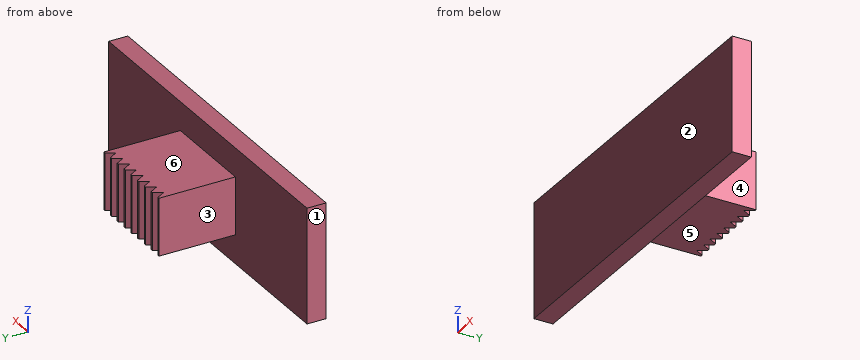
from build123d import *

# Parameters (mm, degrees)
SKETCH1_W           = 18
SKETCH1_H           = 6
BOSS_EXTRUDE1_DEPTH = 1
SKETCH2_W           = 5
SKETCH2_H           = 3
BOSS_EXTRUDE2_DEPTH = 4
CUT_EXTRUDE1_START  = -5.5
CUT_EXTRUDE1_DEPTH  = 8
LPATTERN1_COUNT     = 8
LPATTERN1_PITCH     = 0.614285714


with BuildPart() as part:
    # Sketch1 → Boss-Extrude1 (new body)
    with BuildSketch(Plane(origin=(0, 0, 0), x_dir=(1, 0, 0), z_dir=(0, 1, 0))):
        Rectangle(SKETCH1_W, SKETCH1_H)
    extrude(amount=BOSS_EXTRUDE1_DEPTH)

    # Sketch2 → Boss-Extrude2 (add)
    with BuildSketch(Plane(origin=(0, 1, 0), x_dir=(1, 0, 0), z_dir=(0, 1, 0))):
        Rectangle(SKETCH2_W, SKETCH2_H)
    extrude(amount=BOSS_EXTRUDE2_DEPTH)

    # Sketch3 → Cut-Extrude1 (cut)
    with BuildSketch(Plane.XY.offset(1.5).offset(CUT_EXTRUDE1_START)):
        Polygon((-2.15, 4.566987298), (-1.9, 5), (-2.4, 5), align=None)
    cut_extrude1 = extrude(amount=CUT_EXTRUDE1_DEPTH, mode=Mode.SUBTRACT)

    # LPattern1: Cut-Extrude1 ×8
    with Locations(*[(i * LPATTERN1_PITCH, 0, 0) for i in range(1, LPATTERN1_COUNT)]):
        add(cut_extrude1, mode=Mode.SUBTRACT)


solid = part.part
Geometry check sheet. Reference: the model listing, model coordinates, mm. Face numbers are marked on the shaded views. A direction names the side the tool comes from. Give positions to 0.01 mm unless a question says otherwise; leave off trailing zeros. Loops run counter-clockwise (first coordinate to the right, second up) from the corner with the lowest first, then second, coordinate; pieces in that order, holes last. Notation, with made-up numbers: M 26,35.5 L 42,35.5 A20 cw 42,69.5 Z; hole C 19,85 d6. An arc over 180 degrees is marked long. Write each question's results on one line, items separated by ' | '.
1) Gauge pin test, flat ends, axial feed: pin 1 (1.5 mm diameter, centred on y = 2, z = 0, fed in from +X); pin 2 (1.2 mm diameter, centred on x = -1, y = 4, fed in from +Z); pin 3 (1.2 mm diameter, centred on x = -1, y = 2, fed in from -Z). Record the tip position at first contact, or that the pin passes through.
Answers follow:
pin 1: x = 2.5 | pin 2: z = 1.5 | pin 3: z = -1.5
2) Section check C-C, the plane y = 2. Record the boundary of the cut face in (x, z), plus the area to 3 significant figures.
Answers follow:
outline: M -2.5,-1.5 L 2.5,-1.5 L 2.5,1.5 L -2.5,1.5 Z | area: 15.0 mm2
3) Section check B-B, the plane x = -6.75. Record the boundary of the cut face in (y, z), plus the area to 3 significant figures.
Answers follow:
outline: M 0,-3 L 1,-3 L 1,3 L 0,3 Z | area: 6.00 mm2
4) Thickness scan on line 1 (Z direction, x = 2, y = 1.7); line 2 (Y direction, x = -4, z = -0.45); line 3 (X direction, y = 2.4, z = 0.05). Record the ranges inside material, lowest first.
Answers follow:
line 1: -1.5 to 1.5 | line 2: 0 to 1 | line 3: -2.5 to 2.5
5) Tool access check on the marked faces 3, 4, 5 and 6. Record the directions out of +Z, -Z, +X, -X, +Y, -Y that give a thin tool (end or side, any length) a straight path to the whole face; none if there is none.
Answers follow:
face 3: +Z, -Z, -X, +Y | face 4: +Z, -Z, +X, +Y | face 5: -Z, +X, -X, +Y | face 6: +Z, +X, -X, +Y
6) Release check for a two-part mould opening along Y. For the marked faces 1 and 2 record: +Y half, -Y half, draft (parallel to the pull), parting line (faces both ways), or undercut.
Answers follow:
face 1: draft | face 2: -Y half
